Autodesk Inventor part; units mm, degrees
ref_plane "工作平面1" through (0, 30, 0) normal (0, -1, 0) x (1, 0, 0)
ref_plane "YZ Plane" through (0, 0, 0) normal (1, 0, 0) x (0, 1, 0)
ref_plane "XZ Plane" through (0, 0, 0) normal (0, 1, 0) x (-1, 0, 0)
sketch "草圖1" plane through (0, 0, 0) normal (0, 0, 1) x (1, 0, 0)
  line L0 (0, 30) -> (0, 8)
  line L1 (8, 0) -> (19.6077, 0)
  line L2 (24.8038, -9) -> (15, -25.9808)
  arc A0 (0, 8) -> (8, 0) centre (8, 8) ccw
  arc A1 (24.8038, -9) -> (19.6077, 0) centre (19.6077, -6) ccw
  point P0 (0, 0)
  point P1 (30, 0)
  dimension "d0" = 60
  dimension "d1" = 30
  dimension "d2" = 30
  dimension "d3" = 15
  dimension "d4" = 8
  dimension "d5" = 6
ref_plane "工作平面1" through (0, 30, 0) normal (0, -1, 0) x (1, 0, 0)
sketch "草圖2" plane through (0, 30, 0) normal (0, -1, 0) x (1, 0, 0)
  circle A0 centre (0, 0) radius 4
  dimension "d6" = 8
sweep "掃掠1" add profiles "草圖2" path "草圖1"
properties part number "示範二"
Verification items for the finished model (mm, model axes). Coordinates: 2 decimals unless noted, no trailing zeros. Write each loop counter-clockwise with the first axis right and the second up, starting at its lowest first coordinate (ties: lowest second). Pieces come first, ordered by that corner, then holes. Notation, with made-up numbers: M 24.25,48.5 L 76.25,48.5 A17 ccw 76.25,56.5 Z; hole C 23.25,41.5 d2. An arc over 180 degrees is marked long. One line per item, written item: value.
Item 1: Scan lines: line 1 along Y through (x, z) = (16, -0.75); line 2 along X through (y, z) = (10, 3.5); line 3 along Y through (x, z) = (5.5, -3.5). Record each from-to range of solid material in increasing order.
Check sheet entries:
line 1: y = -26.56 to -16.39, -3.93 to 3.93
line 2: x = -1.94 to 1.94
line 3: y = -1.62 to 2.48
Item 2: Section check A-A, the plane y = 18. Record the boundary of the cut face in (x, z), plus the area to 3 significant figures.
Check sheet entries:
outline: C 0,0 d8
area: 50.3 mm^2
Item 3: Gauge pin test, flat ends, axial feed: pin 1 Ø4 at (x, z) = (22.5, -0.5) entering from -Y; pin 2 Ø2 at (y, z) = (21.5, -2) entering from -X; pin 3 Ø3 at (x, z) = (15.5, 0) entering from +Y. Record the tip position at first contact, or that the pin passes through.
Check sheet entries:
pin 1: stops at y = -24.41
pin 2: stops at x = -3.87
pin 3: stops at y = 4
Item 4: Mould release check, pull along Y, two halves, no side actions. Record for faces 1 (the cylindrical face through (13.885, -0.867, -3.905)), 2 (the cylindrical face through (-0.867, 18.846, -3.905)), 3 (the flat face through (15.05, -26.01, -0.06)): pulls with the +Y half, pulls with the -Y half, needs draft (parallel to the pull), parting line crosses it, or undercut.
Check sheet entries:
face 1: undercut
face 2: needs draft
face 3: pulls with the -Y half
